CAD build for the part. Positions are in the model's coordinates, mm. Coordinates: 2 decimals unless noted, no trailing zeros. Loops run counter-clockwise (first coordinate to the right, second up) from the corner with the lowest first, then second, coordinate; pieces in that order, holes last. Notation, with made-up numbers: (63, -29.75) -> (79, -29.75) arc R19 cw to (79, -21.75) -> close; hole circle Ø5 at (73.25, 28). An arc over 180 degrees is marked (long way). Answer as CSV lines item,"result". Start each with the question number.
Autodesk Inventor part; units mm, degrees
ref_plane "YZ Plane" through (0, 0, 0) normal (1, 0, 0) x (0, 1, 0)
ref_plane "XZ Plane" through (0, 0, 0) normal (0, 1, 0) x (-1, 0, 0)
ref_plane "XY Plane" through (0, 0, 0) normal (0, 0, 1) x (1, 0, 0)
sketch "スケッチ1" plane through (0, 0, 0) normal (0, 0, 1) x (1, 0, 0)
  circle A0 centre (0, 0) radius 18
  dimension "d0" = 36
extrude "押し出し1" add sketch "スケッチ1" along normal blind 3.25
sketch "スケッチ2" plane through (0, 0, 3.25) normal (0, 0, 1) x (1, 0, 0)
  circle A0 centre (0, 0) radius 6
  point P0 (0, 6)
  point P1 (-6, 0)
  point P2 (0, -6)
  point P3 (6, 0)
  dimension "d3" = 12
  dimension "d6" = 360
hole "穴1" at (0, 6, 3.25) at (-6, 0, 3.25) at (0, -6, 3.25) at (6, 0, 3.25) direction (0, 0, -1) diameter 3.2 end through all
sketch "スケッチ3" plane through (0, 0, 0) normal (0, 0, -1) x (-1, 0, 0)
  circle A0 centre (0, 0) radius 8.5
  point P0 (-6.0104, 6.0104)
  point P1 (-6.0104, -6.0104)
  point P2 (6.0104, -6.0104)
  point P3 (6.0104, 6.0104)
  dimension "d15" = 17
  dimension "d18" = 360
hole "穴2" at (6.0104, 6.0104, 0) at (6.0104, -6.0104, 0) at (-6.0104, -6.0104, 0) at (-6.0104, 6.0104, 0) direction (0, 0, 1) diameter 3.2 end through all counterbore diameter 6.5 counterbore depth 10
sketch "スケッチ4" plane through (0, 0, 0) normal (0, 0, -1) x (-1, 0, 0)
  circle A0 centre (0, 0) radius 3.25
  dimension "d27" = 6.5
extrude "押し出し2" cut sketch "スケッチ4" against normal blind 8
sketch "スケッチ5" plane through (0, 0, 3.25) normal (0, 0, 1) x (1, 0, 0)
  circle A0 centre (0, 0) radius 15
  point P0 (0, -15)
  point P1 (10.6066, -10.6066)
  point P2 (15, 0)
  point P3 (10.6066, 10.6066)
  point P4 (0, 15)
  point P5 (-10.6066, 10.6066)
  point P6 (-15, 0)
  point P7 (-10.6066, -10.6066)
  dimension "d31" = 30
  dimension "d34" = 360
hole "穴3" at (0, -15, 3.25) at (10.6066, -10.6066, 3.25) at (15, 0, 3.25) at (10.6066, 10.6066, 3.25) at (0, 15, 3.25) at (-10.6066, 10.6066, 3.25) at (-15, 0, 3.25) at (-10.6066, -10.6066, 3.25) direction (0, 0, -1) diameter 3.2 end through all
sketch "スケッチ7" plane through (0, 0, 3.25) normal (0, 0, 1) x (1, 0, 0)
  circle A0 centre (2.0753, 21.9019) radius 4
  circle A1 centre (-17, 14) radius 4 construction
  circle A2 centre (-3.264, -21.7565) radius 4
  circle A3 centre (0, 0) radius 18
  line L0 (-3.264, -21.7565) -> (0, 0) construction
  circle A4 centre (-20.8592, 6.9924) radius 4 construction
  circle A5 centre (-10.8624, 19.1313) radius 4 construction
  line L1 (-10.8624, 19.1313) -> (0, 0) construction
  line L2 (0, 0) -> (-20.8592, 6.9924) construction
  line L3 (0, 0) -> (2.0753, 21.9019) construction
  arc A6 (-3.8575, -25.7123) -> (2.4526, 25.8841) centre (0, 0) ccw
  circle A7 centre (0, 0) radius 18
  circle A8 centre (-5.8935, 21.1959) radius 4
  circle A9 centre (-10.8278, -19.1509) radius 4
  circle A10 centre (0, 0) radius 22
  point P0 (-1.9091, 21.5489)
  point P1 (-7.1494, -20.8059)
  point P2 (-4.822, 17.3421)
  point P3 (-8.8591, -15.669)
  point P4 (-7.0459, -20.4537)
  point P5 (-1.9247, 21.9156)
  point P6 (-1.9091, 21.5489)
  dimension "d57" = 44
  dimension "d46" = 17
  dimension "d47" = 14
  dimension "d48" = 8
  dimension "d49" = 8
  dimension "d50" = 8
  dimension "d51" = 8
  dimension "d52" = 8
  dimension "d53" = 35
  dimension "d54" = 100
  dimension "d55" = 8
  dimension "d56" = 8
extrude "押し出し4" add sketch "スケッチ7" against normal up to surface (3.25 mm away) contours A10 A2 A3 A0 | A0 A10 | A3 A8 A0 | A2 A10 | A9 A3 A2 picked at (1.947, 20.5476) picked at (-3.0622, -20.4112)
properties part number "s_base6" material "ABS プラスチック"
Q1. Saw through at D-D (y = -5). List the corners of the cut face in (x, z), and give its area (3 significant figures).
Q2. Saw through at C-C (z = 0.6). Give the number of separate pieces and of enclosed holes in the cut face, and give its area (3 significant figures).
Q3. Probe probe 1 along Y at (x, z) = (7, 2.35); probe 2 along Y at (x, z) = (0, 2.3); probe 3 along Y at (x, z) = (-6, 1.25). List the from-to ranges inside material, lowest first. Write a range as from..to.
Q4. Two-plate mould, pull along X, no slides. Class faces 1 (the flat face through (2, -5, 3.25)), 2 (the cylindrical face through (21.764, -3.214, 1.648)), 3 (the cylindrical face through (-12.193, -10.398, 1.602)), 4 (the cylindrical face through (8.9, 7.5, 1.6)): pulls with the +X half, pulls with the -X half, needs draft (parallel to the pull), parting line crosses it, or undercut.
Q5. Saw through at B-B (y = 0). List the corners of the cut face in (x, z), and give its area (3 significant figures).
Q6. Saw through at A-A (x = 0). List the corners of the cut face in (y, z), and give its area (3 significant figures).
Q7. Pin check, flat tip, straight feed: pin 1 Ø1 at (y, z) = (-5.5, 1.5) entering from +X. Stop position of the tip, or through.
Ans:
1,outline,"(-17.29, 0) -> (-9.1, 0) -> (-9.1, 3.25) -> (-17.29, 3.25) -> close; (-2.92, 0) -> (-1.25, 0) -> (-1.25, 3.25) -> (-2.92, 3.25) -> close; (1.25, 0) -> (2.92, 0) -> (2.92, 3.25) -> (1.25, 3.25) -> close; (9.1, 0) -> (21.42, 0) -> (21.42, 3.25) -> (9.1, 3.25) -> close"
1,area,"77.6 mm²"
2,separate pieces,"1"
2,enclosed holes,"17"
2,area,"1,050 mm²"
3,probe 1,"y = -20.86..-9.11, -2.91..-1.25, 1.25..2.91, 9.11..20.86"
3,probe 2,"y = -22..-16.6, -13.4..-7.6, -4.4..-3.25, 3.25..4.4, 7.6..13.4, 16.6..22"
3,probe 3,"y = -21.17..-9.26, -2.76..-1.6, 1.6..2.76, 9.26..16.97"
4,face 1,"needs draft"
4,face 2,"parting line crosses it"
4,face 3,"undercut"
4,face 4,"undercut"
5,outline,"(-18, 0) -> (-16.6, 0) -> (-16.6, 3.25) -> (-18, 3.25) -> close; (-13.4, 0) -> (-7.6, 0) -> (-7.6, 3.25) -> (-13.4, 3.25) -> close; (-4.4, 0) -> (-3.25, 0) -> (-3.25, 3.25) -> (-4.4, 3.25) -> close; (3.25, 0) -> (4.4, 0) -> (4.4, 3.25) -> (3.25, 3.25) -> close; (7.6, 0) -> (13.4, 0) -> (13.4, 3.25) -> (7.6, 3.25) -> close; (16.6, 0) -> (22, 0) -> (22, 3.25) -> (16.6, 3.25) -> close"
5,area,"67.3 mm²"
6,outline,"(-22, 0) -> (-16.6, 0) -> (-16.6, 3.25) -> (-22, 3.25) -> close; (-13.4, 0) -> (-7.6, 0) -> (-7.6, 3.25) -> (-13.4, 3.25) -> close; (-4.4, 0) -> (-3.25, 0) -> (-3.25, 3.25) -> (-4.4, 3.25) -> close; (3.25, 0) -> (4.4, 0) -> (4.4, 3.25) -> (3.25, 3.25) -> close; (7.6, 0) -> (13.4, 0) -> (13.4, 3.25) -> (7.6, 3.25) -> close; (16.6, 0) -> (22, 0) -> (22, 3.25) -> (16.6, 3.25) -> close"
6,area,"80.3 mm²"
7,pin 1,"stops at x = 21.42"
